```python
from build123d import *

# Parameters (mm, degrees)
SKETCH1_W               = 8
SKETCH1_H               = 5
BOSS_EXTRUDE1_DEPTH     = 2
BOSS_EXTRUDE2_DEPTH     = 5
BOSS_EXTRUDE5_DEPTH     = 2
CUT_EXTRUDE2_DEPTH      = 1
CUT_EXTRUDE2_DEPTH_BACK = 6


with BuildPart() as part:
    # Sketch1 → Boss-Extrude1 (new body)
    with BuildSketch(Plane.XY):
        with Locations((-17, 0)):
            Rectangle(SKETCH1_W, SKETCH1_H)
    extrude(amount=BOSS_EXTRUDE1_DEPTH)

    # Sketch2 → Boss-Extrude2 (add)
    with BuildSketch(Plane(origin=(0, 0, 0), x_dir=(-1, 0, 0), z_dir=(0, 0, -1))):
        with BuildLine():
            Line((21, 2.5), (17.320508076, 2.5))
            ThreePointArc((17.320508076, 2.5), (17.5, 0), (17.320508076, -2.5))
            Line((17.320508076, -2.5), (21, -2.5))
            Line((21, -2.5), (21, 2.5))
        make_face()
    extrude(amount=BOSS_EXTRUDE2_DEPTH)

    # Sketch3 → Boss-Extrude5 (add)
    with BuildSketch(Plane(origin=(0, 0, -5), x_dir=(-1, 0, 0), z_dir=(0, 0, -1))):
        with BuildLine():
            Line((21, 2.5), (17.320508076, 2.5))
            ThreePointArc((17.320508076, 2.5), (17.5, 0), (17.320508076, -2.5))
            Line((17.320508076, -2.5), (21, -2.5))
            Line((21, -2.5), (21, 2.5))
        make_face()
        with BuildLine():
            Line((17.320508076, 2.5), (13, 2.5))
            Line((13, 2.5), (13, -2.5))
            Line((13, -2.5), (17.320508076, -2.5))
            ThreePointArc((17.320508076, -2.5), (17.5, 0), (17.320508076, 2.5))
        make_face()
    extrude(amount=BOSS_EXTRUDE5_DEPTH)

    # Sketch4 → Cut-Extrude2 (cut, two sides)
    with BuildSketch(Plane(origin=(0, 2.5, 0), x_dir=(1, 0, 0), z_dir=(0, 1, 0))) as cut_extrude2_sk:
        with BuildLine():
            Line((-13, 0), (-15.006873144, 0))
            ThreePointArc((-15.006873144, 0), (-13.924543455, -0.231950336), (-13, -0.840602876))
            Line((-13, -0.840602876), (-13, 0))
        make_face()
        with BuildLine():
            ThreePointArc((-17.320508076, -1), (-16.343812237, -0.276562376), (-15.160254038, 0))
            Line((-15.160254038, 0), (-17.320508076, 0))
            Line((-17.320508076, 0), (-17.320508076, -1))
        make_face()
    extrude(amount=CUT_EXTRUDE2_DEPTH, mode=Mode.SUBTRACT)
    extrude(cut_extrude2_sk.sketch, amount=-CUT_EXTRUDE2_DEPTH_BACK, mode=Mode.SUBTRACT)


solid = part.part
```
Part model, mm, in its own coordinate system. A direction names the side the tool comes from. Round coordinates to 2 decimals unless told otherwise and drop trailing zeros. Write each loop counter-clockwise with the first axis right and the second up, starting at its lowest first coordinate (ties: lowest second). Pieces come first, ordered by that corner, then holes. Notation, with made-up numbers: (67.25, -16.5) -> (77.25, -16.5) arc R12 cw to (77.25, 1.5) -> close; hole circle Ø2 at (20, 10.25). An arc over 180 degrees is marked (long way). Return JSON: item names as keys, results as strings. Group by question number.
Q1. Mould opens along Z. For faces 1 (the flat face through (-13, 0, 1)), 2 (the flat face through (-17.321, 0, 0.5)), 3 (the flat face through (-17, 0, 2)) say: pulls with the +Z half, pulls with the -Z half, needs draft (parallel to the pull), parting line crosses it, or undercut.
Q2. Which spindle directions (+Z, -Z, +X, -X, +Y, -Y) get a long thin tool onto all of the face, cutting with end or side? Do faces 4 (the cylindrical face through (-17.5, 0, -2.5)), 5 (the cylindrical face through (-13.939, 0.035, 0.226)), 6 (the flat face through (-18, 2.5, -2)). Say none if no direction does.
Q3. Saw through at A-A on x = -17. Write the cut outline in (y, z), plus the area to 3 significant figures.
Q4. Saw through at D-D on z = -3.25. Write the cut outline in (x, y).
Q5. Pin check, flat tips, straight feed: pin 1 (0.5 mm diameter, centred on y = -0.5, z = 0.5, fed in from +X); pin 2 (4 mm diameter, centred on x = -17, z = 0.5, fed in from +Y). Stop position of each tip, or through.
Q6. Probe L1, parallel to Z at x = -15, y = 0.4; L2, parallel to Z at x = -13.5, y = -0.8; L3, parallel to X at y = 1.45, z = -4. List the from-to ranges inside material, lowest first. Write a range as [from, to].
Q7. Saw through at B-B on z = 0.5. Write the cut outline in (x, y).
Q8. Saw through at C-C on y = -1.45. Write the cut outline in (x, z).
Answer:
{
 "1": {"face 1": "needs draft", "face 2": "undercut", "face 3": "pulls with the +Z half"},
 "2": {"face 4": "+X", "face 5": "+X, +Y, -Y", "face 6": "+Z, -Z, +X, -X, +Y"},
 "3": {"outline": "(-2.5, -7) -> (2.5, -7) -> (2.5, -5) -> (-2.5, -5) -> close; (-2.5, 0.69) -> (2.5, 0.69) -> (2.5, 2) -> (-2.5, 2) -> close", "area": "16.5 mm2"},
 "4": {"outline": "(-21, -2.5) -> (-17.32, -2.5) arc R17.5 cw to (-17.32, 2.5) -> (-21, 2.5) -> close"},
 "5": {"pin 1": "x = -13.1", "pin 2": "y = 2.5"},
 "6": {"L1": "[-7, -5], [0, 2]", "L2": "[-7, -5], [0.45, 2]", "L3": "[-21, -17.44]"},
 "7": {"outline": "(-21, -2.5) -> (-17.32, -2.5) -> (-17.32, 2.5) -> (-21, 2.5) -> close; (-16.74, -2.5) -> (-13.42, -2.5) -> (-13.42, 2.5) -> (-16.74, 2.5) -> close"},
 "8": {"outline": "(-21, -7) -> (-13, -7) -> (-13, -5) -> (-17.44, -5) -> (-17.44, 0) -> (-17.32, 0) -> (-17.32, 1) arc R3 ccw to (-15.16, 0) -> (-15.01, 0) arc R3 ccw to (-13, 0.84) -> (-13, 2) -> (-21, 2) -> close"}
}
